Can you work these out from the model? Positions are in its coordinate system, mm. Give positions to 0.01 mm unless a question says otherwise; leave off trailing zeros. Order: outer loops, then holes, each group sorted by start corner. A loop starts at its lowest first (then second) coordinate and runs counter-clockwise, first axis right, second up. Notation, with made-up numbers: M 54,-36.75 L 62,-36.75 A14 ccw 62,-26.75 Z; hole C 44.5,26 d11. An arc over 180 degrees is marked long. Use a Markdown table: item, result. Add a question column.
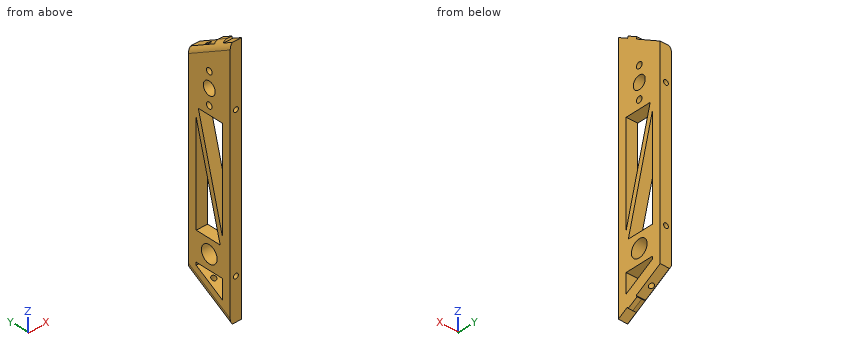
from build123d import *

# Parameters (mm, degrees)
SKETCH1_R                     = 3.6195
SKETCH1_R_2                   = 4.7625
SKETCH1_R_3                   = 1.6999966
BOSS_EXTRUDE1_DEPTH           = 6.35
TAP_DRILL_FOR_6_32_TAP4_D     = 2.7051
TAP_DRILL_FOR_6_32_TAP4_DEPTH = 10.16
TAP_DRILL_FOR_6_32_TAP4_TIP   = 0.81269403
TAP_DRILL_FOR_6_32_TAP3_D     = 2.7051
TAP_DRILL_FOR_6_32_TAP3_DEPTH = 10.16
TAP_DRILL_FOR_6_32_TAP3_TIP   = 0.81269403
SKETCH11_W                    = 6.35
SKETCH11_H                    = 6.1722
BOSS_EXTRUDE2_DEPTH           = 1.016
SKETCH12_W                    = 6.35
SKETCH12_H                    = 6.1722
BOSS_EXTRUDE3_DEPTH           = 1.016
TAP_DRILL_FOR_6_32_TAP1_D     = 2.7051
TAP_DRILL_FOR_6_32_TAP1_DEPTH = 7.62
TAP_DRILL_FOR_6_32_TAP1_TIP   = 0.81269403
TAP_DRILL_FOR_6_32_TAP2_D     = 2.7051
TAP_DRILL_FOR_6_32_TAP2_DEPTH = 7.62
TAP_DRILL_FOR_6_32_TAP2_TIP   = 0.81269403
CUT_EXTRUDE1_DEPTH            = 143.132235964
FILLET1_R                     = 3.81


with BuildPart() as part:
    # Sketch1 → Boss-Extrude1 (new body)
    with BuildSketch(Plane(origin=(0, 0, 0), x_dir=(0, 0, -1), z_dir=(1, 0, 0))):
        Polygon((0, 0), (-14.664696837, 25.4), (-125.035303163, 25.4), (-139.7, 0), align=None)
        with Locations((-110.998, 12.7)):
            Circle(SKETCH1_R, mode=Mode.SUBTRACT)
        with Locations((-28.702, 12.7)):
            Circle(SKETCH1_R_2, mode=Mode.SUBTRACT)
        with Locations((-102.4979916, 12.7)):
            Circle(SKETCH1_R_3, mode=Mode.SUBTRACT)
        with Locations((-119.4980084, 12.7)):
            Circle(SKETCH1_R_3, mode=Mode.SUBTRACT)
    extrude(amount=BOSS_EXTRUDE1_DEPTH)

    # Tap Drill for #6-32 Tap4
    with Locations(Plane(origin=(0, 25.4, 0), x_dir=(1, 0, 0), z_dir=(0, 1, 0))):
        with Locations((3.175, -105.985303163), (3.175, -34.984696837)):
            Hole(TAP_DRILL_FOR_6_32_TAP4_D / 2, depth=TAP_DRILL_FOR_6_32_TAP4_DEPTH)
            with Locations((0, 0, -(TAP_DRILL_FOR_6_32_TAP4_DEPTH + TAP_DRILL_FOR_6_32_TAP4_TIP / 2))):  # 118° drill point
                Cone(0, TAP_DRILL_FOR_6_32_TAP4_D / 2, TAP_DRILL_FOR_6_32_TAP4_TIP, mode=Mode.SUBTRACT)

    # Tap Drill for #6-32 Tap3
    with Locations(Plane(origin=(0, 0, 0), x_dir=(-1, 0, 0), z_dir=(0, -1, 0))):
        with Locations((-3.175, -105.41), (-3.175, -22.86)):
            Hole(TAP_DRILL_FOR_6_32_TAP3_D / 2, depth=TAP_DRILL_FOR_6_32_TAP3_DEPTH)
            with Locations((0, 0, -(TAP_DRILL_FOR_6_32_TAP3_DEPTH + TAP_DRILL_FOR_6_32_TAP3_TIP / 2))):  # 118° drill point
                Cone(0, TAP_DRILL_FOR_6_32_TAP3_D / 2, TAP_DRILL_FOR_6_32_TAP3_TIP, mode=Mode.SUBTRACT)

    # Sketch11 → Boss-Extrude2 (add)
    with BuildSketch(Plane(origin=(0, 60.491874454, 104.775), x_dir=(1, 0, 0), z_dir=(0, 0.5000000000000037, 0.8660254037844365))):
        with Locations((3.175, -60.4139)):
            Rectangle(SKETCH11_W, SKETCH11_H)
    extrude(amount=BOSS_EXTRUDE2_DEPTH)

    # Sketch12 → Boss-Extrude3 (add)
    with BuildSketch(Plane(origin=(0, 0, 0), x_dir=(-1, 0, 0), z_dir=(0, 0.49999999999999806, -0.8660254037844398))):
        with Locations((-3.175, 9.4361)):
            Rectangle(SKETCH12_W, SKETCH12_H)
    extrude(amount=BOSS_EXTRUDE3_DEPTH)

    # Tap Drill for #6-32 Tap1
    with Locations(Plane(origin=(0, 60.491874454, 104.775), x_dir=(1, 0, 0), z_dir=(0, 0.5000000000000037, 0.8660254037844365))):
        with Locations((3.175, -50.680606325)):
            Hole(TAP_DRILL_FOR_6_32_TAP1_D / 2, depth=TAP_DRILL_FOR_6_32_TAP1_DEPTH)
            with Locations((0, 0, -(TAP_DRILL_FOR_6_32_TAP1_DEPTH + TAP_DRILL_FOR_6_32_TAP1_TIP / 2))):  # 118° drill point
                Cone(0, TAP_DRILL_FOR_6_32_TAP1_D / 2, TAP_DRILL_FOR_6_32_TAP1_TIP, mode=Mode.SUBTRACT)

    # Tap Drill for #6-32 Tap2
    with Locations(Plane(origin=(0, 0, 0), x_dir=(-1, 0, 0), z_dir=(0, 0.49999999999999806, -0.8660254037844398))):
        with Locations((-3.175, 19.169393675)):
            Hole(TAP_DRILL_FOR_6_32_TAP2_D / 2, depth=TAP_DRILL_FOR_6_32_TAP2_DEPTH)
            with Locations((0, 0, -(TAP_DRILL_FOR_6_32_TAP2_DEPTH + TAP_DRILL_FOR_6_32_TAP2_TIP / 2))):  # 118° drill point
                Cone(0, TAP_DRILL_FOR_6_32_TAP2_D / 2, TAP_DRILL_FOR_6_32_TAP2_TIP, mode=Mode.SUBTRACT)

    # Sketch19 → Cut-Extrude1 (cut, through all)
    with BuildSketch(Plane.ZY):
        Polygon((92.68551049, 20.6375), (36.6395, 20.6375), (36.6395, 6.07467201), align=None)
        Polygon((97.7354916, 4.7625), (97.7354916, 19.32532799), (41.68948111, 4.7625), align=None)
        Polygon((20.7645, 20.6375), (20.7645, 4.7625), (10.081979076, 4.7625), (19.247414599, 20.6375), align=None)
    extrude(amount=-CUT_EXTRUDE1_DEPTH, mode=Mode.SUBTRACT)

    # Fillet1
    fillet1_edges = [part.edges().sort_by_distance(p)[0] for p in [
        (0, 8.679902313, 135.86183181),
        (0, 8.679902313, 3.83816819),
    ]]
    fillet(fillet1_edges, radius=FILLET1_R)


solid = part.part
1. If we section it at B-B, the plane z = 12: State how many separate pieces and enclosed holes the cut face has, then the cut area to 3 significant figures.
2. Will these pins go through, and if not, where does the flat tip stop? pin 1 (2.5 mm diameter, centred on x = 3.18, z = 105.99, fed in from +Y); pin 2 (1 mm diameter, centred on x = 4, y = 12, fed in from +Z).
3. I need wall thicknesses on L1, parallel to Z at x = 2.25, y = 2.75; L2, parallel to Y at x = 3.75, z = 12; L3, parallel to X at y = 5.75, z = 22.86. Which ranges of each line are inside material? Lowest first, please. Write a range as [from, to].
4. If we section it at A-A, the plane z = 86.5: List the corners of the cut face in (x, y) for me, then the cut area to 3 significant figures.
Geometry results:
| question | item | result |
|---|---|---|
| 1 | separate pieces | 2 |
| 1 | enclosed holes | 1 |
| 1 | area | 102 mm^2 |
| 2 | pin 1 | stops at y = 15.18 |
| 2 | pin 2 | stops at z = 133.06 |
| 3 | L1 | z = [1.59, 21.87], [23.85, 104.42], [106.4, 138.11] |
| 3 | L2 | y = [0, 4.76], [8.08, 13.79], [16.62, 20.78] |
| 3 | L3 | x = [0, 1.82], [4.53, 6.35] |
| 4 | outline | M 0,0 L 6.35,0 L 6.35,4.76 L 0,4.76 Z; M 0,16.41 L 6.35,16.41 L 6.35,19.03 L 0,19.03 Z; M 0,20.64 L 6.35,20.64 L 6.35,25.4 L 0,25.4 Z |
| 4 | area | 77.1 mm^2 |
